Here's how the part is built. I have some questions about the finished solid (model axes, mm). A direction names the side the tool comes from. Round coordinates to 2 decimals unless told otherwise and drop trailing zeros. Write each loop counter-clockwise with the first axis right and the second up, starting at its lowest first coordinate (ties: lowest second). Pieces come first, ordered by that corner, then holes. Notation, with made-up numbers: (45.5, 45.5) -> (95.5, 45.5) arc R4 ccw to (95.5, 50.5) -> close; hole circle Ø10 at (-26, 54.25). An arc over 180 degrees is marked (long way). Answer in a Markdown table with one row per item.
Autodesk Inventor part; units mm, degrees
ref_plane "YZ Plane" through (0, 0, 0) normal (1, 0, 0) x (0, 1, 0)
ref_plane "XZ Plane" through (0, 0, 0) normal (0, 1, 0) x (-1, 0, 0)
ref_plane "XY Plane" through (0, 0, 0) normal (0, 0, 1) x (1, 0, 0)
sketch "Эскиз1" plane through (0, 0, 0) normal (0, 1, 0) x (-1, 0, 0)
  line L0 (0, 24) -> (20, 24)
  line L1 (20, 24) -> (20, 0)
  line L2 (20, 0) -> (0, 0)
  line L3 (20, 24) -> (14, 24)
  line L4 (14, 16) -> (6, 16)
  line L5 (20, 0) -> (-20, 0)
  line L6 (-20, 0) -> (-20, 16)
  line L7 (-20, 16) -> (0, 16)
  line L8 (-20, 0) -> (-20, 12.5)
  line L9 (0, 16) -> (0, 24)
  line L10 (10, 24) -> (3.5, 24)
  line L11 (3.5, 24) -> (6, 16)
  line L12 (3.5, 24) -> (16.5, 24)
  line L13 (16.5, 24) -> (14, 16)
  line L14 (20, 0) -> (20, 16.5)
  line L15 (0, 0) -> (5, 0)
  line L16 (0, 16) -> (5, 16)
  line L17 (-20, 12.5) -> (5, 12.5)
  line L18 (5, 12.5) -> (20, 12.5)
  point P0 (16.5, 24)
  point P1 (20, 20.5)
  dimension "d0" = 24
  dimension "d1" = 20
  dimension "d3" = 8
  dimension "d5" = 40
  dimension "d6" = 16
  dimension "d7" = 12.5
  dimension "d15" = 6.5
  dimension "d16" = 13
revolve "Вращение4" add sketch "Эскиз1" angle 360 about axis through (-20, 0, 0) along (1, 0, 0) contours L0 L11 L4 L13 L1 L18 L17 L6 L7 L9
sketch "Эскиз4" plane through (0, 0, 0) normal (0, 1, 0) x (-1, 0, 0)
  line L0 (-20, 16) -> (-20, -16)
  line L1 (-20, 0) -> (0, 0)
  line L2 (0, 0) -> (-10, 0)
  circle A0 centre (-10, 0) radius 1.5
  dimension "d43" = 3
extrude "Выдавливание5" cut sketch "Эскиз4" along normal mid plane 59.25
thread "Резьба4"
properties part number "17701729.303661.004"
1) We'd pull the mould along Y, two halves only. Please class faces 1 (the face through (-0.28, 3.755, 11.923)), 2 (the face through (9.86, -15.62, -3.47)), 3 (the face through (11.5, -14.18, 0.07)): +Y half, -Y half, draft (parallel to the pull), parting line (faces both ways), or undercut.
Response:
| item | result |
|---|---|
| face 1 | undercut |
| face 2 | parting line |
| face 3 | draft |
2) I want a section at B-B, the plane z = 0. List the corners of the cut face in (x, y) for me, and give its area (3 significant figures).
Response:
| item | result |
|---|---|
| outline | (-20, -24) -> (-16.5, -24) -> (-14, -16) -> (-6, -16) -> (-3.5, -24) -> (0, -24) -> (0, -16) -> (8.5, -16) -> (8.5, -12.5) -> (-20, -12.5) -> close; (-20, 12.5) -> (8.5, 12.5) -> (8.5, 16) -> (0, 16) -> (0, 24) -> (-3.5, 24) -> (-6, 16) -> (-14, 16) -> (-16.5, 24) -> (-20, 24) -> close; (11.5, -16) -> (20, -16) -> (20, -12.5) -> (11.5, -12.5) -> close; (11.5, 12.5) -> (20, 12.5) -> (20, 16) -> (11.5, 16) -> close |
| area | 411 mm^2 |
3) I want a section at A-A, the plane y = 0. List the corners of the cut face in (x, z) for me.
Response:
| item | result |
|---|---|
| outline | (-20, -24) -> (-16.5, -24) -> (-14, -16) -> (-6, -16) -> (-3.5, -24) -> (0, -24) -> (0, -16) -> (20, -16) -> (20, -12.5) -> (-20, -12.5) -> close; (-20, 12.5) -> (20, 12.5) -> (20, 16) -> (0, 16) -> (0, 24) -> (-3.5, 24) -> (-6, 16) -> (-14, 16) -> (-16.5, 24) -> (-20, 24) -> close |
4) I need wall thicknesses on line 1 (Y direction, x = -7.5, z = 0); line 2 (X direction, y = 14, z = 0). Which ranges of each line are inside material? Lowest first, please. Write a range as [from, to].
Response:
| item | result |
|---|---|
| line 1 | y = [-16, -12.5], [12.5, 16] |
| line 2 | x = [-20, 8.5], [11.5, 20] |
5) Which directions (+Z, -Z, +X, -X, +Y, -Y) give clear straight access to the entire face, cutting with the end or side of a thin tool? Please do faces 4 (the face through (11.5, 14.18, -0.07)), 5 (the face through (-5.844, 16.108, -3.577)), 6 (the face through (0, 16, 5)).
Response:
| item | result |
|---|---|
| face 4 | +Y, -Y |
| face 5 | none |
| face 6 | +X |
6) I want a section at D-D, the plane x = -12.5. List the corners of the cut face in (y, z) for me.
Response:
| item | result |
|---|---|
| outline | circle Ø32 at (0, 0); hole circle Ø25 at (0, 0) |
7) I want a section at C-C, the plane x = 10. List the corners of the cut face in (y, z) for me, and give its area (3 significant figures).
Response:
| item | result |
|---|---|
| outline | (-15.93, -1.5) arc R16 ccw to (15.93, -1.5) -> (12.41, -1.5) arc R12.5 cw to (-12.41, -1.5) -> close; (-15.93, 1.5) -> (-12.41, 1.5) arc R12.5 cw to (12.41, 1.5) -> (15.93, 1.5) arc R16 ccw to start |
| area | 292 mm^2 |
8) For pin 1 (5 mm diameter, centred on x = -5.5, z = -8, fed in from -Y); pin 2 (3.5 mm diameter, centred on x = 10, z = 0, fed in from +Y); pin 3 (3 mm diameter, centred on x = -10, y = -11, fed in from +Z), each with a flat end and sliding along its axis, tell me the tip position at first contact or that it passes through.
Response:
| item | result |
|---|---|
| pin 1 | stops at y = -23.1 |
| pin 2 | stops at y = 16 |
| pin 3 | stops at z = 12.87 |
